Build history of the part. All positions in model axes, mm. Face numbers are marked on the shaded views. A direction names the side the tool comes from. Round coordinates to 2 decimals unless told otherwise and drop trailing zeros. Write each loop counter-clockwise with the first axis right and the second up, starting at its lowest first coordinate (ties: lowest second). Pieces come first, ordered by that corner, then holes.
1) Wall check: probe 1 along Y at (x, z) = (0, 70.5); probe 2 along Z at (x, y) = (2.25, 0.25); probe 3 along Z at (x, y) = (-0.5, 8). Give the ranges that are in metal, low to high.
2) Flat gauge pins, fed straight in: pin 1 (3 mm diameter, centred on y = -5.5, z = 43.5, fed in from +X); pin 2 (11 mm diameter, centred on x = 1, z = 6.5, fed in from +Y); pin 3 (12 mm diameter, centred on x = -7.5, z = 59, fed in from +Y). Where does each tip first touch, or does it go through?
3) Saw through at B-B (x = 11). Write the cut outline in (y, z).
4) Saw through at C-C (x = -7.5). Write the cut outline in (y, z).
5) Pull direction Z, two halves, no side cores. Call the marked faces 1, 2, 3 and 4: +Z half, -Z half, draft (parallel to the pull), parting line (faces both ways), or undercut.
6) Saw through at A-A (z = 6). Write the cut outline in (x, y).
7) Which spindle directions (+Z, -Z, +X, -X, +Y, -Y) get a long thin tool onto all of the face, cutting with end or side? Do the marked faces 5, 6 and 7. Say none if no direction does.
8) Saw through at D-D (z = 22.5). Write the cut outline in (x, y).
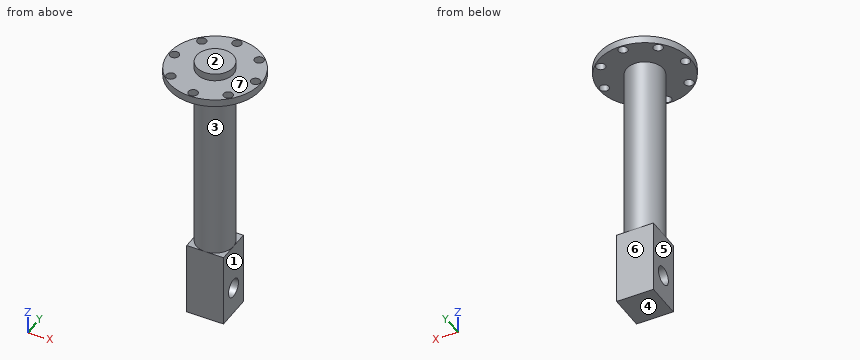
from build123d import *

# Parameters (mm, degrees)
SKIZZE1_W                       = 10
SKIZZE1_H                       = 10
AUFSATZ_LINEAR_AUSTRAGEN1_DEPTH = 20
SKIZZE2_R                       = 2.5
SCHNITT_LINEAR_AUSTRAGEN1_DEPTH = 20
SKIZZE3_R                       = 5
AUFSATZ_LINEAR_AUSTRAGEN2_DEPTH = 50
SKIZZE4_R                       = 12.5
AUFSATZ_LINEAR_AUSTRAGEN3_DEPTH = 2
SKIZZE5_R                       = 1.25
SCHNITT_LINEAR_AUSTRAGEN2_DEPTH = 5
SKIZZE6_R                       = 5
AUFSATZ_LINEAR_AUSTRAGEN4_DEPTH = 2


with BuildPart() as part:
    # Skizze1 → Aufsatz-Linear austragen1 (new body)
    with BuildSketch(Plane.XY):
        Rectangle(SKIZZE1_W, SKIZZE1_H)
    extrude(amount=AUFSATZ_LINEAR_AUSTRAGEN1_DEPTH)

    # Skizze2 → Schnitt-Linear austragen1 (cut)
    with BuildSketch(Plane(origin=(5, 0, 0), x_dir=(0, 0, -1), z_dir=(1, 0, 0))):
        with Locations(Location((-7.5, 0, 0), (0, 0, 90))):
            Circle(SKIZZE2_R)
    extrude(amount=-SCHNITT_LINEAR_AUSTRAGEN1_DEPTH, mode=Mode.SUBTRACT)

    # Skizze3 → Aufsatz-Linear austragen2 (add)
    with BuildSketch(Plane.XY.offset(20)):
        Circle(SKIZZE3_R)
    extrude(amount=AUFSATZ_LINEAR_AUSTRAGEN2_DEPTH)

    # Skizze4 → Aufsatz-Linear austragen3 (add)
    with BuildSketch(Plane.XY.offset(70)):
        Circle(SKIZZE4_R)
    extrude(amount=AUFSATZ_LINEAR_AUSTRAGEN3_DEPTH)

    # Skizze5 → Schnitt-Linear austragen2 (cut)
    with BuildSketch(Plane.XY.offset(72)):
        with Locations((0, 11)):
            Circle(SKIZZE5_R)
        with Locations((7.778174593, 7.778174593)):
            Circle(SKIZZE5_R)
        with Locations((11, 0)):
            Circle(SKIZZE5_R)
        with Locations((7.778174593, -7.778174593)):
            Circle(SKIZZE5_R)
        with Locations((0, -11)):
            Circle(SKIZZE5_R)
        with Locations((-7.778174593, -7.778174593)):
            Circle(SKIZZE5_R)
        with Locations((-11, 0)):
            Circle(SKIZZE5_R)
        with Locations((-7.778174593, 7.778174593)):
            Circle(SKIZZE5_R)
    extrude(amount=-SCHNITT_LINEAR_AUSTRAGEN2_DEPTH, mode=Mode.SUBTRACT)

    # Skizze6 → Aufsatz-Linear austragen4 (add)
    with BuildSketch(Plane.XY.offset(72)):
        Circle(SKIZZE6_R)
    extrude(amount=AUFSATZ_LINEAR_AUSTRAGEN4_DEPTH)


solid = part.part
Evaluation:
1. probe 1: y = -12.5 to -12.25, -9.75 to 9.75, 12.25 to 12.5
1. probe 2: z = 0 to 5.01, 9.99 to 74
1. probe 3: z = 70 to 72
2. pin 1: stops at x = 3
2. pin 2: stops at y = 5
2. pin 3: stops at y = 4.77
3. outline: (-5.94, 70) - (-1.25, 70) - (-1.25, 72) - (-5.94, 72) - close; (1.25, 70) - (5.94, 70) - (5.94, 72) - (1.25, 72) - close
4. outline: (-10, 70) - (-9, 70) - (-9, 72) - (-10, 72) - close; (-6.56, 70) - (6.56, 70) - (6.56, 72) - (-6.56, 72) - close; (9, 70) - (10, 70) - (10, 72) - (9, 72) - close
5. face 1: draft
5. face 2: +Z half
5. face 3: undercut
5. face 4: -Z half
6. outline: (-5, -5) - (5, -5) - (5, -2) - (-5, -2) - close; (-5, 2) - (5, 2) - (5, 5) - (-5, 5) - close
7. face 5: -Z, -X, +Y, -Y
7. face 6: -Z, +X, -X, +Y
7. face 7: +Z
8. outline: circle Ø10 at (0, 0)
